Job drawing, mm, ordinate dimensions from the low corner. One solid piece. A direction names the side the tool comes from. Give positions to 0.01 mm unless a question says otherwise; leave off trailing zeros. Loops run counter-clockwise (first coordinate to the right, second up) from the corner with the lowest first, then second, coordinate; pieces in that order, holes last. Notation, with made-up numbers: M 37,59 L 42,59 A29 cw 42,79 Z; hole C 20,-20.75 d4. An arc over 180 degrees is marked long. Put each result on its own line as item: value.
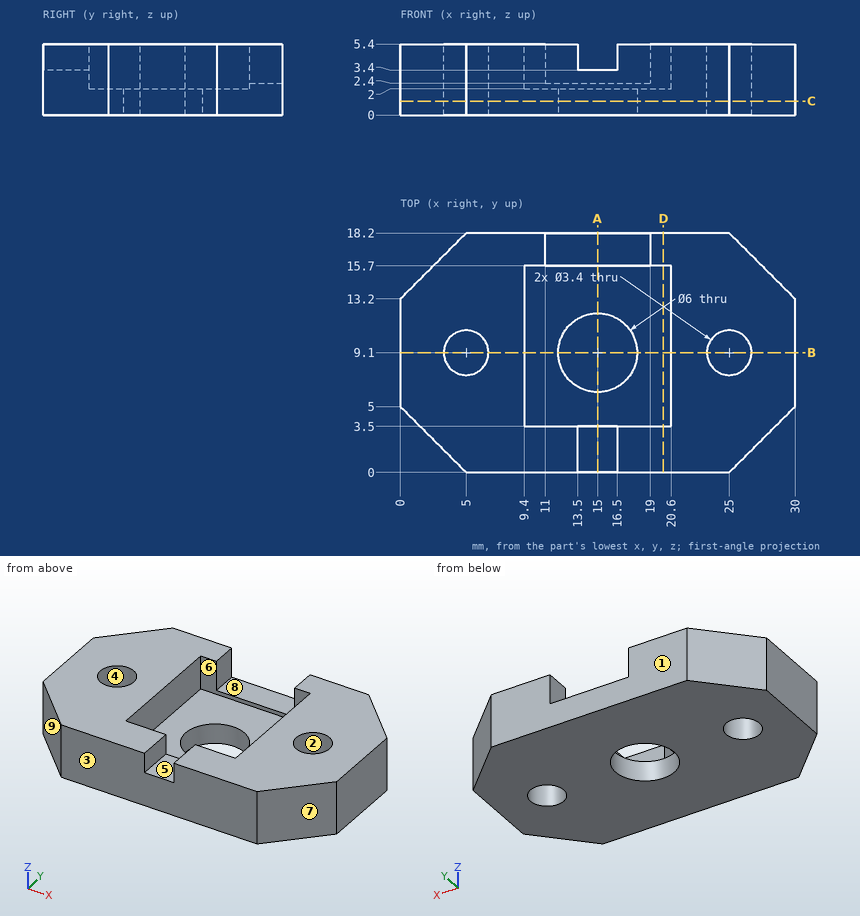
Q1. Tool access for the marked faces 5, 6, 7, 8 and 9: list every direction of +Z, -Z, +X, -X, +Y, -Y with a clear straight run to the whole face (end or side of a thin tool).
Here are the results:
face 5: +Z, +Y, -Y
face 6: +Z
face 7: +Z, -Z, +X, -Y
face 8: +Z, +Y
face 9: +Z, -Z, -X, -Y
Q2. Slice it at C-C (z = 1.05). List the corners of the cut face in (x, y), and give its area (3 significant figures).
Here are the results:
outline: M 0,5 L 5,0 L 25,0 L 30,5 L 30,13.2 L 25,18.2 L 5,18.2 L 0,13.2 Z; hole C 5,9.1 d3.4; hole C 15,9.1 d6; hole C 25,9.1 d3.4
area: 450 mm²
Q3. Mould opens along Y. For the marked faces 1, 2, 3 and 4 say: pulls with the +Y half, pulls with the -Y half, needs draft (parallel to the pull), parting line crosses it, or undercut.
Here are the results:
face 1: pulls with the +Y half
face 2: undercut
face 3: pulls with the -Y half
face 4: undercut
Q4. Slice it at B-B (y = 9.1). List the corners of the cut face in (x, z).
Here are the results:
outline: M 0,0 L 3.3,0 L 3.3,5.4 L 0,5.4 Z; M 6.7,0 L 12,0 L 12,2 L 9.4,2 L 9.4,5.4 L 6.7,5.4 Z; M 18,0 L 23.3,0 L 23.3,5.4 L 20.6,5.4 L 20.6,2 L 18,2 Z; M 26.7,0 L 30,0 L 30,5.4 L 26.7,5.4 Z
Q5. Slice it at D-D (x = 20). List the corners of the cut face in (y, z).
Here are the results:
outline: M 0,0 L 18.2,0 L 18.2,5.4 L 15.7,5.4 L 15.7,2 L 3.5,2 L 3.5,5.4 L 0,5.4 Z
Q6. Slice it at A-A (x = 15). List the corners of the cut face in (y, z).
Here are the results:
outline: M 0,0 L 6.1,0 L 6.1,2 L 3.5,2 L 3.5,3.4 L 0,3.4 Z; M 12.1,0 L 18.2,0 L 18.2,2.4 L 15.7,2.4 L 15.7,2 L 12.1,2 Z
Q7. Drop flat-ended pins along their axis: pin 1 Ø0.8 at (y, z) = (16.5, 3) entering from +X; pin 2 Ø1.5 at (x, y) = (14.5, 2) entering from +Z; pin 3 Ø3.5 at (x, y) = (13, 9.5) entering from +Z. Give the stop position or say it passes through.
Here are the results:
pin 1: x = 27.1
pin 2: z = 3.4
pin 3: z = 2
Q8. Probe line 1 (X direction, y = 9.1, z = 1); line 2 (X direction, y = 9.1, z = 4); line 3 (Y direction, x = 25, z = 2.85). List the from-to ranges inside material, lowest first. Write a range as from..to.
Here are the results:
line 1: 0..3.3, 6.7..12, 18..23.3, 26.7..30
line 2: 0..3.3, 6.7..9.4, 20.6..23.3, 26.7..30
line 3: 0..7.4, 10.8..18.2
